Can you work these out from the model? Positions are in its coordinate system, mm. Face numbers are marked on the shaded views. A direction names the side the tool comes from. Give positions to 0.01 mm unless a question says otherwise; leave off trailing zeros. Loops run counter-clockwise (first coordinate to the right, second up) from the corner with the lowest first, then second, coordinate; pieces in that order, holes last. Notation, with made-up numbers: (33.5, -33) - (70.5, -33) arc R8 cw to (70.5, -28) - close; hole circle Ø1 at (14.25, 35.25). An arc over 180 degrees is marked (long way). Write item = value, one per line.
from build123d import *

# Parameters (mm, degrees)
BOSS_EXTRUDE1_DEPTH = 15.5
CUT_EXTRUDE1_DEPTH  = 24
CUT_EXTRUDE2_DEPTH  = 13.5
CUT_EXTRUDE3_DEPTH  = 13.5
CUT_EXTRUDE4_DEPTH  = 13.5
SKETCH6_R           = 1.15
CUT_EXTRUDE5_DEPTH  = 10.5
SKETCH8_W           = 5
SKETCH8_H           = 2
CUT_EXTRUDE7_DEPTH  = 5.5
SKETCH9_W           = 5
SKETCH9_H           = 2
CUT_EXTRUDE8_DEPTH  = 5.5
SKETCH10_W          = 5
SKETCH10_H          = 2
CUT_EXTRUDE9_DEPTH  = 5.5
CUT_EXTRUDE10_DEPTH = 20
BOSS_EXTRUDE2_DEPTH = 13.5
BOSS_EXTRUDE3_DEPTH = 13.5
SKETCH15_R          = 1.25
CUT_EXTRUDE11_DEPTH = 8.5
SKETCH19_W          = 17
SKETCH19_H          = 2
CUT_EXTRUDE15_DEPTH = 13.5
CUT_EXTRUDE16_DEPTH = 10
CUT_EXTRUDE17_DEPTH = 5.7
CUT_EXTRUDE18_DEPTH = 5.7
CUT_EXTRUDE19_DEPTH = 5.7


with BuildPart() as part:
    # Sketch1 → Boss-Extrude1 (new body)
    with BuildSketch(Plane(origin=(0, 0, 0), x_dir=(1, 0, 0), z_dir=(0, 1, 0))):
        Polygon((127, 0), (-63.5, 109.985226281), (-63.5, -109.985226281), align=None)
    extrude(amount=BOSS_EXTRUDE1_DEPTH)

    # Sketch2 → Cut-Extrude1 (cut)
    with BuildSketch(Plane(origin=(0, 15.5, 0), x_dir=(1, 0, 0), z_dir=(0, 1, 0))):
        Polygon((-63.5, -109.985226281), (16.5, -63.797204745), (-63.5, -17.60918321), align=None)
        Polygon((-63.5, 109.985226281), (16.5, 63.797204745), (-63.5, 17.60918321), align=None)
        Polygon((127, 0), (47, 46.188021535), (47, -46.188021535), align=None)
    extrude(amount=-CUT_EXTRUDE1_DEPTH, mode=Mode.SUBTRACT)

    # Sketch3 → Cut-Extrude2 (cut)
    with BuildSketch(Plane(origin=(0, 15.5, 0), x_dir=(1, 0, 0), z_dir=(0, 1, 0))):
        Polygon((21, 28.217265235), (21, 13.217265235), (16.2, 13.217265235), (16.2, 11.217265235), (21, 11.217265235), (21, 8.217265235), (27, 8.217265235), (27, 0), (45, 0), (46, 0), (46, 21.217265235), (46, 25.017265235), (45, 25.017265235), (45, 28.217265235), align=None)
        Polygon((14.186868519, -31.862153395), (1.196487462, -24.362153395), (3.596487462, -20.205231457), (1.864436654, -19.205231457), (-0.535563346, -23.362153395), (-3.133639557, -21.862153395), (-6.133639557, -27.058305818), (-13.25, -22.9496732), (-22.25, -38.538130468), (-23, -39.837168574), (-4.625309308, -50.445801192), (-1.334412773, -52.345801192), (-0.584412773, -51.046763086), (2.186868519, -52.646763086), align=None)
        Polygon((-35.28503876, 3.29953441), (-22.294657703, 10.79953441), (-19.894657703, 6.642612472), (-17.564436654, 7.987966222), (-19.964436654, 12.14488816), (-17.366360443, 13.64488816), (-20.616360443, 19.274053285), (-13.5, 23.382685902), (-22.5, 38.97114317), (-23, 39.837168574), (-41.374690692, 29.228535957), (-45.263757468, 26.983182207), (-44.513757468, 25.684144101), (-47.28503876, 24.084144101), align=None)
    extrude(amount=-CUT_EXTRUDE2_DEPTH, mode=Mode.SUBTRACT)

    # Sketch4 → Cut-Extrude3 (cut)
    with BuildSketch(Plane(origin=(0, 15.5, 0), x_dir=(1, 0, 0), z_dir=(0, 1, 0))):
        Polygon((3.668919326, -54.079775788), (16.5, -61.487803669), (35, -50.806823689), (45, -33.486315613), (45, -5.916079783), (46, 0), (44, 0), (44, -2), (25, -2), (25, 6.217265235), (19, 6.217265235), (19, 9.217265235), (14.2, 9.217265235), (14.2, 15.217265235), (19, 15.217265235), (19, 30.217265235), (45, 30.217265235), (45, 45.033320997), (26.5, 55.714300977), (6.5, 55.714300977), (-15.626136458, 42.939770137), (-23, 39.837168574), (-22, 38.105117767), (-20.267949192, 39.105117767), (-10.767949192, 22.650635095), (-17.884309636, 18.542002477), (-14.634309636, 12.912837353), (-17.232385847, 11.412837353), (-14.832385847, 7.255915414), (-20.626708511, 3.910561665), (-23.026708511, 8.067483603), (-36.017089568, 0.567483603), (-49.267089568, 23.517156803), (-61.5, 16.454482672), (-61.5, -4.907477288), (-51.5, -22.227985364), (-27.623475383, -36.013103279), (-23, -39.837168574), (-22, -38.105117767), (-23.732050808, -37.105117767), (-13.982050808, -20.217622393), (-6.865690364, -24.32625501), (-3.865690364, -19.130102587), (-1.267614153, -20.630102587), (1.132385847, -16.473180649), (6.32853827, -19.473180649), (3.92853827, -23.630102587), (16.918919326, -31.130102587), align=None)
    extrude(amount=-CUT_EXTRUDE3_DEPTH, mode=Mode.SUBTRACT)

    # Sketch5 → Cut-Extrude4 (cut)
    with BuildSketch(Plane(origin=(0, 2, 0), x_dir=(1, 0, 0), z_dir=(0, 1, 0))):
        Polygon((14.43375673, 0), (7.216878365, 12.5), (-7.216878365, 12.5), (-14.43375673, 0), (-7.216878365, -12.5), (7.216878365, -12.5), align=None)
    extrude(amount=-CUT_EXTRUDE4_DEPTH, mode=Mode.SUBTRACT)

    # Sketch6 → Cut-Extrude5 (cut)
    with BuildSketch(Plane(origin=(0, 15.5, 0), x_dir=(1, 0, 0), z_dir=(0, 1, 0))):
        with Locations((-59.125, -15.083275783)):
            Circle(SKETCH6_R)
        with Locations((16.5, 58.74538989)):
            Circle(SKETCH6_R)
        with Locations((42.625, -43.662114107)):
            Circle(SKETCH6_R)
    extrude(amount=-CUT_EXTRUDE5_DEPTH, mode=Mode.SUBTRACT)

    # Sketch8 → Cut-Extrude7 (cut)
    with BuildSketch(Plane(origin=(-48.25, 0, 27.857150488), x_dir=(-0.5, 0, -0.866025404), z_dir=(0.866025404, 0, -0.5))):
        with Locations((16.5, 5.1)):
            Rectangle(SKETCH8_W, SKETCH8_H)
    extrude(amount=-CUT_EXTRUDE7_DEPTH, mode=Mode.SUBTRACT)

    # Sketch9 → Cut-Extrude8 (cut)
    with BuildSketch(Plane(origin=(48.25, 0, 27.857150488), x_dir=(-0.5, 0, 0.866025404), z_dir=(-0.866025404, 0, -0.5))):
        with Locations((16.5, 5.1)):
            Rectangle(SKETCH9_W, SKETCH9_H)
    extrude(amount=-CUT_EXTRUDE8_DEPTH, mode=Mode.SUBTRACT)

    # Sketch10 → Cut-Extrude9 (cut)
    with BuildSketch(Plane.XY.offset(-55.714300977)):
        with Locations((16.5, 5.1)):
            Rectangle(SKETCH10_W, SKETCH10_H)
    extrude(amount=-CUT_EXTRUDE9_DEPTH, mode=Mode.SUBTRACT)

    # Sketch12 → Cut-Extrude10 (cut)
    with BuildSketch(Plane(origin=(0, 15.5, 0), x_dir=(1, 0, 0), z_dir=(0, 1, 0))):
        Polygon((-49.267089568, 23.517156803), (-49.267089568, -25.82655788), (-63.5, -17.60918321), (-63.5, 17.60918321), (-49.267089568, 25.82655788), align=None)
        Polygon((3.668919326, -54.079775788), (47, -29.062564697), (47, -46.188021535), (16.5, -63.797204745), (1.668919326, -55.234476326), align=None)
        Polygon((45, 30.217265235), (0, 54.270925304), (16.5, 63.797204745), (47, 46.188021535), (47, 29.062564697), align=None)
    extrude(amount=-CUT_EXTRUDE10_DEPTH, mode=Mode.SUBTRACT)

    # Sketch13 → Boss-Extrude2 (add)
    with BuildSketch(Plane(origin=(0, 2, 0), x_dir=(1, 0, 0), z_dir=(0, 1, 0))):
        Polygon((-49.267089568, -23.517156803), (-49.267089568, 23.517156803), (-47.267089568, 20.053055188), (-47.267089568, -24.671857341), align=None)
        Polygon((45, -30.217265235), (3.668919326, -54.079775788), (5.668919326, -50.615674173), (45, -27.907864158), align=None)
        Polygon((45, 30.217265235), (2.07703105, 53.160698663), (0.037424254, 51.98313113), (40.757379657, 30.217265235), align=None)
    extrude(amount=BOSS_EXTRUDE2_DEPTH)

    # Sketch14 → Boss-Extrude3 (add)
    with BuildSketch(Plane(origin=(0, 2, 0), x_dir=(1, 0, 0), z_dir=(0, 1, 0))):
        Polygon((-47.267089568, -24.671857341), (-36.767089568, -30.734035168), (-47.267089568, -12.547501688), align=None)
        Polygon((0.037424254, 51.98313113), (-10.462575746, 45.920953304), (10.730086226, 46.267627657), align=None)
        Polygon((45, -27.907864158), (45, -15.783508505), (34.5, -33.970041985), align=None)
    extrude(amount=BOSS_EXTRUDE3_DEPTH)

    # Sketch15 → Cut-Extrude11 (cut)
    with BuildSketch(Plane(origin=(0, 15.5, 0), x_dir=(1, 0, 0), z_dir=(0, 1, 0))):
        with Locations((-44.615165779, -23.140768428)):
            Circle(SKETCH15_R)
        with Locations((42.348076211, -26.376775245)):
            Circle(SKETCH15_R)
        with Locations((0.06687762, 49.09429048)):
            Circle(SKETCH15_R)
    extrude(amount=-CUT_EXTRUDE11_DEPTH, mode=Mode.SUBTRACT)

    # Sketch19 → Cut-Extrude15 (cut)
    with BuildSketch(Plane(origin=(0, 15.5, 0), x_dir=(1, 0, 0), z_dir=(0, 1, 0))):
        Polygon((-13.25, -22.9496732), (-22, -38.105117767), (-23.732050808, -37.105117767), (-14.982050808, -21.9496732), align=None)
        Polygon((-13.5, 23.382685902), (-22, 38.105117767), (-20.267949192, 39.105117767), (-11.767949192, 24.382685902), align=None)
        with Locations((35.5, -1)):
            Rectangle(SKETCH19_W, SKETCH19_H)
    extrude(amount=-CUT_EXTRUDE15_DEPTH, mode=Mode.SUBTRACT)

    # Sketch20 → Cut-Extrude16 (cut)
    with BuildSketch(Plane(origin=(0, 15.5, 0), x_dir=(1, 0, 0), z_dir=(0, 1, 0))):
        Polygon((46, 0), (45.5, -2.958039892), (47, -2.958039892), (47, 0), (47, 6), (46, 6), align=None)
        Polygon((-23, 39.837168574), (-28.196152423, 36.837168574), (-28.696152423, 37.703193978), (-23.5, 40.703193978), (-20.063068229, 42.687507461), (-19.313068229, 41.388469355), align=None)
        Polygon((-23, -39.837168574), (-17.803847577, -42.837168574), (-18.303847577, -43.703193978), (-23.5, -40.703193978), (-26.061737691, -39.224174032), (-25.311737691, -37.925135926), align=None)
    extrude(amount=-CUT_EXTRUDE16_DEPTH, mode=Mode.SUBTRACT)

    # Sketch16 → Cut-Extrude17 (cut)
    with BuildSketch(Plane(origin=(-0.753783321, 0, -46.079771924), x_dir=(0.999866231, 0, -0.016356038), z_dir=(0.016356038, 0, 0.999866231))):
        Polygon((-1.612342698, 12.5), (0.887657302, 13.5), (3.387657302, 12.5), (3.387657302, 10), (-1.612342698, 10), align=None)
    extrude(amount=-CUT_EXTRUDE17_DEPTH, mode=Mode.SUBTRACT)

    # Sketch17 → Cut-Extrude18 (cut)
    with BuildSketch(Plane(origin=(-40.883544784, 0, 23.604125586), x_dir=(-0.5, 0, -0.866025404), z_dir=(0.866025404, 0, -0.5))):
        Polygon((-0.232910432, 12.5), (-0.232910432, 9.5), (4.767089568, 9.5), (4.767089568, 12.5), (2.267089568, 13.5), align=None)
    extrude(amount=-CUT_EXTRUDE18_DEPTH, mode=Mode.SUBTRACT)

    # Sketch18 → Cut-Extrude19 (cut)
    with BuildSketch(Plane(origin=(40.584459663, 0, 23.431448711), x_dir=(-0.5, 0, 0.866025404), z_dir=(-0.866025404, 0, -0.5))):
        Polygon((-0.831080674, 12.5), (-0.831080674, 9.5), (4.168919326, 9.5), (4.168919326, 12.5), (1.668919326, 13.5), align=None)
    extrude(amount=-CUT_EXTRUDE19_DEPTH, mode=Mode.SUBTRACT)


solid = part.part
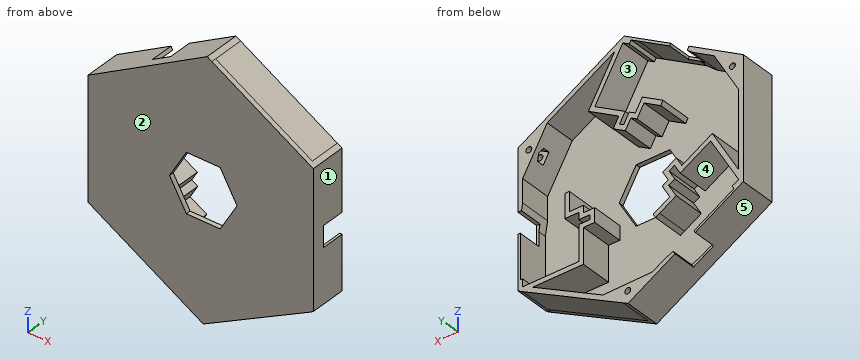
Q1. Imagine slicing it at A-A, the plane z = 9. Write out the boundary of the cut face in (x, y).
Output:
outline = (-49.27, 0) - (-9.24, 0) - (-9.24, 2) - (-47.27, 2) - (-47.27, 15.5) - (-49.27, 15.5) - close; (9.24, 0) - (47, 0) - (47, 15.5) - (45, 15.5) - (45, 2) - (9.24, 2) - close
Q2. We'd pull the mould along X, two halves only. Please class the marked faces 1, 2 and 3: released by +X, released by -X, zero draft, split by the parting line, or undercut.
Output:
face_1 = released by +X
face_2 = zero draft
face_3 = undercut
Q3. Imagine slicing it at B-B, the plane y = 11.25. Give the number of separate pieces and of enclosed holes in the cut face, then the cut area to 3 significant figures.
Output:
separate_pieces = 3
enclosed_holes = 0
area = 1,060 mm2
Q4. For pin 1 (1.2 mm diameter, centred on x = 46, z = 0, fed in from +Y); pin 2 (4 mm diameter, centred on x = 19.5, y = 11.5, fed in from +Z); pin 3 (4 mm diameter, centred on y = 3.5, z = 39, fed in from +X), each with a flat end and sliding along its axis, tell me the tip position at first contact or that it passes through.
Output:
pin_1 = 5.5
pin_2 = 46.09
pin_3 = 33.25
Q5. Imagine slicing it at D-D, the plane x = 37. Write out the boundary of the cut face in (y, z), then the cut area to 3 significant figures.
Output:
outline = (0, -34.49) - (15.5, -34.49) - (15.5, -32.23) - (2, -32.23) - (2, -30.22) - (15.5, -30.22) - (15.5, -28.22) - (2, -28.22) - (2, 29.64) - (15.5, 29.64) - (15.5, 34.84) - (0, 34.84) - close
area = 266 mm2
Q6. Which directions (+Z, -Z, +X, -X, +Y, -Y) give clear straight access to the entire face, cutting with the end or side of a thin tool? Please do the marked faces 4 and 5.
Output:
face_4 = +Y
face_5 = -Z, -X, +Y, -Y
Q7. Imagine slicing it at C-C, the plane x = -38. Write out the boundary of the cut face in (y, z).
Output:
outline = (0, -32.33) - (15.5, -32.33) - (15.5, -31.18) - (2, -31.18) - (2, -8) - (15.5, -8) - (15.5, -4) - (2, -4) - (2, 28.6) - (15.5, 28.6) - (15.5, 32.33) - (0, 32.33) - close
Q8. I need wall thicknesses on L1, parallel to X at y = 4.5, z = -0.5; L2, parallel to X at y = 13.75, z = -21; L3, parallel to X at y = 14.5, z = -2. Which ranges of each line are inside material? Lowest first, please.
Output:
L1 = -49.27 to -47.27, 25 to 27, 46 to 47
L2 = -49.27 to -45.5, -17.63 to -13.63, 19 to 21, 46 to 47
L3 = -49.27 to -47.27, -36.84 to -33.54, 25 to 27
